from build123d import *

# Parameters (mm, degrees)
SKETCH_1_W          = 58
SKETCH_1_H          = 25.4
EXTRUDE_1_DEPTH     = 3
SKETCH_2_W          = 8
SKETCH_2_H          = 3
EXTRUDE_2_DEPTH     = 28
SKETCH_3_R          = 3
CUT_EXTRUDE_1_DEPTH = 12
SKETCH_4_R          = 2
CUT_EXTRUDE_2_DEPTH = 22
SKETCH_8_W          = 8
SKETCH_8_H          = 3
CUT_EXTRUDE_3_DEPTH = 28


with BuildPart() as part:
    # 草图1 → 凸台-拉伸1 (new body)
    with BuildSketch(Plane(origin=(0, 0, 0), x_dir=(1, 0, 0), z_dir=(0, 1, 0))):
        Rectangle(SKETCH_1_W, SKETCH_1_H)
    extrude(amount=EXTRUDE_1_DEPTH)

    # 草图2 → 凸台-拉伸2 (add)
    with BuildSketch(Plane(origin=(0, 3, 0), x_dir=(1, 0, 0), z_dir=(0, 1, 0))):
        with Locations((-24.75, 11.2)):
            Rectangle(SKETCH_2_W, SKETCH_2_H)
        with Locations((24.75, 11.2)):
            Rectangle(SKETCH_2_W, SKETCH_2_H)
        with Locations((-24.75, 0)):
            Rectangle(SKETCH_2_W, SKETCH_2_H)
        with Locations((24.75, 0)):
            Rectangle(SKETCH_2_W, SKETCH_2_H)
    extrude(amount=EXTRUDE_2_DEPTH)

    # 草图3 → 切除-拉伸1 (cut, symmetric)
    with BuildSketch(Plane.XY.offset(-9.7)):
        with Locations((-24.75, 12)):
            Circle(SKETCH_3_R)
        with Locations((-24.75, 22)):
            Circle(SKETCH_3_R)
        with Locations((24.75, 12)):
            Circle(SKETCH_3_R)
        with Locations((24.75, 22)):
            Circle(SKETCH_3_R)
    extrude(amount=CUT_EXTRUDE_1_DEPTH, both=True, mode=Mode.SUBTRACT)

    # 草图4 → 切除-拉伸2 (cut)
    with BuildSketch(Plane(origin=(0, 3, 0), x_dir=(1, 0, 0), z_dir=(0, 1, 0))):
        with Locations((24.75, -7.5)):
            Circle(SKETCH_4_R)
        with Locations((24.75, 7.5)):
            Circle(SKETCH_4_R)
        with Locations((-4.85, 7.5)):
            Circle(SKETCH_4_R)
        with Locations((-4.85, -7.5)):
            Circle(SKETCH_4_R)
    extrude(amount=-CUT_EXTRUDE_2_DEPTH, mode=Mode.SUBTRACT)

    # 草图8 → 切除-拉伸3 (cut)
    with BuildSketch(Plane(origin=(0, 31, 0), x_dir=(1, 0, 0), z_dir=(0, 1, 0))):
        with Locations((-24.75, 11.2)):
            Rectangle(SKETCH_8_W, SKETCH_8_H)
        with Locations((24.75, 11.2)):
            Rectangle(SKETCH_8_W, SKETCH_8_H)
    extrude(amount=-CUT_EXTRUDE_3_DEPTH, mode=Mode.SUBTRACT)


solid = part.part
For this review, take the finished solid that the model builds, in its own axes (mm). A direction names the side the tool comes from. Give positions to 0.01 mm unless a question says otherwise; leave off trailing zeros. Loops run counter-clockwise (first coordinate to the right, second up) from the corner with the lowest first, then second, coordinate; pieces in that order, holes last. Notation, with made-up numbers: M -7,53.25 L 14,53.25 A27 ccw 14,80.25 Z; hole C -14,80.25 d1. An arc over 180 degrees is marked long. Answer as a JSON object with one key per item and string values. Group by question number.
Q1. Add section D-D on z = -7.5. Give the boundary of the cut face in (x, y).
Q2. Add section A-A on y = 26. Give the boundary of the cut face in (x, z).
Q3. Mouldability with a two-part tool opening along X and no side actions: class faces 4 (the flat face through (28.75, 17, 0)), 5 (the flat face through (-20.75, 17, 0)), 6 (the flat face through (-25, 17, -1.5)), 7 (the cylindrical face through (21.753, 12.132, -0.021)) as +X half, -X half, draft (parallel to the pull), parting line (faces both ways), or undercut.
Q4. For probe 1 along Y at (x, z) = (-24.75, 0.15); probe 2 along X at (y, z) = (12, -0.4); probe 3 along Z at (x, y) = (-4.85, 2.1), list the stretches that pass through material, from the lowest coordinate up. Write a range as [from, to].
Q5. Add section C-C on y = 22. Give the boundary of the cut face in (x, z), and give its area (3 significant figures).
Q6. Insertion check: P1, Ø1.5, axis at y = 22, z = 0.5, coming from the +X side; P2, Ø9.5, axis at x = -24.75, y = 12, coming from the +Z side; P3, Ø0.9, axis at y = 14, z = -0.5, coming from the -X side. Each pin has a flat end and moves straight along its axis. Give the tip position at first contact, or say it passes through.
Q7. Add section B-B on x = 24.75. Give the boundary of the cut face in (y, z), and give its area (3 significant figures).
Q8. Tool access review of faces 1 (the flat face through (0, 1, 12.7)), 2 (the flat face through (25, 17, 1.5)), 3 (the flat face through (25, 17, -1.5)): name each direction out of +Z, -Z, +X, -X, +Y, -Y from which nothing blocks a thin tool from reaching the whole face with its end or side.
Checked values:
{
 "1": {"outline": "M -29,0 L -6.85,0 L -6.85,3 L -29,3 Z; M -2.85,0 L 22.75,0 L 22.75,3 L -2.85,3 Z; M 26.75,0 L 29,0 L 29,3 L 26.75,3 Z"},
 "2": {"outline": "M -28.75,-1.5 L -20.75,-1.5 L -20.75,1.5 L -28.75,1.5 Z; M 20.75,-1.5 L 28.75,-1.5 L 28.75,1.5 L 20.75,1.5 Z"},
 "3": {"face 4": "+X half", "face 5": "undercut", "face 6": "draft", "face 7": "undercut"},
 "4": {"probe 1": "[0, 9], [15, 19], [25, 31]", "probe 2": "[-28.75, -27.75], [-21.75, -20.75], [20.75, 21.75], [27.75, 28.75]", "probe 3": "[-12.7, -9.5], [-5.5, 5.5], [9.5, 12.7]"},
 "5": {"outline": "M -28.75,-1.5 L -27.75,-1.5 L -27.75,1.5 L -28.75,1.5 Z; M -21.75,-1.5 L -20.75,-1.5 L -20.75,1.5 L -21.75,1.5 Z; M 20.75,-1.5 L 21.75,-1.5 L 21.75,1.5 L 20.75,1.5 Z; M 27.75,-1.5 L 28.75,-1.5 L 28.75,1.5 L 27.75,1.5 Z", "area": "12.0 mm²"},
 "6": {"P1": "x = 28.75", "P2": "z = 1.5", "P3": "x = -28.75"},
 "7": {"outline": "M 0,-12.7 L 3,-12.7 L 3,-9.5 L 0,-9.5 Z; M 0,-5.5 L 3,-5.5 L 3,-1.5 L 9,-1.5 L 9,1.5 L 3,1.5 L 3,5.5 L 0,5.5 Z; M 0,9.5 L 3,9.5 L 3,12.7 L 0,12.7 Z; M 15,-1.5 L 19,-1.5 L 19,1.5 L 15,1.5 Z; M 25,-1.5 L 31,-1.5 L 31,1.5 L 25,1.5 Z", "area": "100 mm²"},
 "8": {"face 1": "+Z, +X, -X, +Y, -Y", "face 2": "+Z, +X, -X, +Y", "face 3": "-Z, +X, -X, +Y"}
}
